Geometry: final body of the model. Coordinates: model frame, mm. A direction names the side the tool comes from. Coordinates: 2 decimals unless noted, no trailing zeros. Write each loop counter-clockwise with the first axis right and the second up, starting at its lowest first coordinate (ties: lowest second). Pieces come first, ordered by that corner, then holes. Notation, with made-up numbers: (20, 2.25) -> (51, 2.25) arc R19 cw to (51, 12.25) -> close; hole circle Ø4 at (77.5, 82.5). An arc over 180 degrees is marked (long way). Answer as a JSON object with one key per item and string values. Group by question number.
```python
from build123d import *

# Parameters (mm, degrees)
F0_W          = 22
F0_H          = 42
F1_DEPTH      = 3
F2_W          = 3
F2_H          = 30
F2_W_2        = 5
F3_DEPTH      = 22
F4_D          = 4.1
F7_DEPTH      = 5
F8_DEPTH      = 2.97
F9_R          = 4.99999
F11_D         = 4.1
F12_D         = 2.8
F13_W         = 22
F13_H         = 10.5
F14_DEPTH     = 8
F15_T1_DEPTH  = 8
F15_T3_DEPTH  = 18
F15_T5_DEPTH  = 18
F15_T7_DEPTH  = 22.7901994578
F15_T9_DEPTH  = 23
F15_T11_DEPTH = 23
F15_T13_DEPTH = 23
F16_D         = 29
F17_D         = 3.1


# Not quite as in the source:
# - a fillet or chamfer that OpenCascade refuses, or shapes differently, is made with other operations: its cross-section is extruded or revolved along the edge and cut away or added
# - a fillet or chamfer is up to 0.001 mm smaller than in the source, because OpenCascade refuses the exact size


with BuildPart() as f1:
    # F0 (on Front) → F1 (new body)
    with BuildSketch(Plane.XZ):
        with Locations((-28.9233987555, 27.9422005266)):
            Rectangle(F0_W, F0_H)
    extrude(amount=F1_DEPTH)

    # F2 (on face) → F3 (join)
    with BuildSketch(Plane(origin=(-39.9233987555, 0, 0), x_dir=(0, -1, 0), z_dir=(-1, 0, 0))):
        with Locations((1.5, 33.9422005266)):
            Rectangle(F2_W, F2_H)
        with Locations((5.5, 33.9422005266)):
            Rectangle(F2_W_2, F2_H)
    extrude(amount=-F3_DEPTH)

    # F4 (through all)
    with Locations(Plane(origin=(0, 0, 0), x_dir=(1, 0, 0), z_dir=(0, 1, 0))):
        with Locations((-24.9233987555, -12.9422005266), (-32.9233987555, -12.9422005266), (-32.9233987555, -32.9422005266), (-24.9233987555, -32.9422005266)):
            Hole(F4_D / 2)

    # F6 (on line) → F7 (join, symmetric)
    with BuildSketch(Plane.XY.offset(23.9422005266)):
        with BuildLine():
            ThreePointArc((-36.9233987555, -20), (-28.9233987555, -12), (-20.9233987555, -20))
            Line((-20.9233987555, -20), (-20.9233987555, -32))
            Line((-20.9233987555, -32), (-17.9233987555, -32))
            Line((-17.9233987555, -32), (-17.9233987555, 0))
            Line((-17.9233987555, 0), (-39.9233987555, 0))
            Line((-39.9233987555, 0), (-39.9233987555, -32))
            Line((-39.9233987555, -32), (-36.9233987555, -32))
            Line((-36.9233987555, -32), (-36.9233987555, -20))
        make_face()
    extrude(amount=F7_DEPTH, both=True)

    # F6 (on line) → F8 (join, symmetric)
    with BuildSketch(Plane.XY.offset(23.9422005266)):
        with BuildLine():
            ThreePointArc((-34.9233987555, -20), (-28.9233987555, -14), (-22.9233987555, -20))
            Line((-22.9233987555, -20), (-22.9233987555, -25.2915026221))
            ThreePointArc((-22.9233987555, -25.2915026221), (-21.4400839819, -22.8284271247), (-20.9233987555, -20))
            ThreePointArc((-20.9233987555, -20), (-28.9233987555, -12), (-36.9233987555, -20))
            ThreePointArc((-36.9233987555, -20), (-36.406713529, -22.8284271247), (-34.9233987555, -25.2915026221))
            Line((-34.9233987555, -25.2915026221), (-34.9233987555, -20))
        make_face()
        with BuildLine():
            Line((-34.9233987555, -32), (-34.9233987555, -25.2915026221))
            ThreePointArc((-34.9233987555, -25.2915026221), (-36.406713529, -22.8284271247), (-36.9233987555, -20))
            Line((-36.9233987555, -20), (-36.9233987555, -32))
            Line((-36.9233987555, -32), (-34.9233987555, -32))
        make_face()
        with BuildLine():
            ThreePointArc((-20.9233987555, -20), (-21.4400839819, -22.8284271247), (-22.9233987555, -25.2915026221))
            Line((-22.9233987555, -25.2915026221), (-22.9233987555, -32))
            Line((-22.9233987555, -32), (-20.9233987555, -32))
            Line((-20.9233987555, -32), (-20.9233987555, -20))
        make_face()
    extrude(amount=F8_DEPTH, both=True)

    # F9 (radius 5 in the source; OpenCascade refuses exactly that, so slightly less here)
    f9_edges = [f1.edges().sort_by_distance(p)[0] for p in [
        (-38.423399, -32, 28.942201),
        (-38.423399, -32, 18.942201),
        (-19.423399, -32, 18.942201),
        (-19.423399, -32, 28.942201),
    ]]
    fillet(f9_edges, radius=F9_R)

    # F11 (through all)
    with Locations(Plane(origin=(-39.9233987555, 0, 0), x_dir=(0, -1, 0), z_dir=(-1, 0, 0))):
        with Locations((4, 44.9422005266), (4, 24.9422005266)):
            Hole(F11_D / 2)

    # F12 (through all)
    with Locations(Plane(origin=(-39.9233987555, 0, 0), x_dir=(0, -1, 0), z_dir=(-1, 0, 0))):
        with Locations((27.5, 23.9422005266)):
            Hole(F12_D / 2)

    # F13 (on Front) → F14 (join)
    with BuildSketch(Plane.XZ):
        Polygon((-57.4233987555, 59.4422005266), (-39.9233987555, 59.4422005266), (-17.9233987555, 59.4422005266), (-15.4233987555, 59.4422005266), (-15.4233987555, 101.4422005266), (-57.4233987555, 101.4422005266), align=None)
        with Locations((-28.9233987555, 54.1922005266)):
            Rectangle(F13_W, F13_H)
    extrude(amount=F14_DEPTH)

    # F15: fillet of radius 3 on 7 edges, made by hand

    # F15_s2 → F15_t1 (join)
    with BuildSketch(Plane.XZ):
        with BuildLine():
            ThreePointArc((-39.9233987555, 56.4422005266), (-40.8020784119, 58.5635208702), (-42.9233987555, 59.4422005266))
            Line((-42.9233987555, 59.4422005266), (-39.9233987555, 59.4422005266))
            Line((-39.9233987555, 59.4422005266), (-39.9233987555, 56.4422005266))
        make_face()
    extrude(amount=F15_T1_DEPTH)

    # F15_s4 → F15_t3 (cut)
    with BuildSketch(Plane.XZ.offset(-7.5)):
        with BuildLine():
            ThreePointArc((-39.9233987555, 9.9422005266), (-39.0447190991, 7.820880183), (-36.9233987555, 6.9422005266))
            Line((-36.9233987555, 6.9422005266), (-39.9233987555, 6.9422005266))
            Line((-39.9233987555, 6.9422005266), (-39.9233987555, 9.9422005266))
        make_face()
    extrude(amount=F15_T3_DEPTH, mode=Mode.SUBTRACT)

    # F15_s6 → F15_t5 (cut)
    with BuildSketch(Plane.XZ.offset(-7.5)):
        with BuildLine():
            ThreePointArc((-17.9233987555, 9.9422005266), (-18.8020784119, 7.820880183), (-20.9233987555, 6.9422005266))
            Line((-20.9233987555, 6.9422005266), (-17.9233987555, 6.9422005266))
            Line((-17.9233987555, 6.9422005266), (-17.9233987555, 9.9422005266))
        make_face()
    extrude(amount=F15_T5_DEPTH, mode=Mode.SUBTRACT)

    # F15_s8 → F15_t7 (cut)
    with BuildSketch(Plane.XZ.offset(-7.3950997289)):
        with BuildLine():
            ThreePointArc((-17.9233987555, 59.4422005266), (-16.132110908, 60.463748745), (-15.4233987555, 62.4002404181))
            Line((-15.4233987555, 62.4002404181), (-15.4233987555, 59.4422005266))
            Line((-15.4233987555, 59.4422005266), (-17.9233987555, 59.4422005266))
        make_face()
    extrude(amount=F15_T7_DEPTH, mode=Mode.SUBTRACT)

    # F15_s10 → F15_t9 (cut)
    with BuildSketch(Plane.XZ.offset(-7.5)):
        with BuildLine():
            ThreePointArc((-18.4233987555, 101.4422005266), (-16.3020784119, 100.5635208702), (-15.4233987555, 98.4422005266))
            Line((-15.4233987555, 98.4422005266), (-15.4233987555, 101.4422005266))
            Line((-15.4233987555, 101.4422005266), (-18.4233987555, 101.4422005266))
        make_face()
    extrude(amount=F15_T9_DEPTH, mode=Mode.SUBTRACT)

    # F15_s12 → F15_t11 (cut)
    with BuildSketch(Plane.XZ.offset(-7.5)):
        with BuildLine():
            ThreePointArc((-57.4233987555, 98.4422005266), (-56.5447190991, 100.5635208702), (-54.4233987555, 101.4422005266))
            Line((-54.4233987555, 101.4422005266), (-57.4233987555, 101.4422005266))
            Line((-57.4233987555, 101.4422005266), (-57.4233987555, 98.4422005266))
        make_face()
    extrude(amount=F15_T11_DEPTH, mode=Mode.SUBTRACT)

    # F15_s14 → F15_t13 (cut)
    with BuildSketch(Plane.XZ.offset(-7.5)):
        with BuildLine():
            ThreePointArc((-54.4233987555, 59.4422005266), (-56.5447190991, 60.320880183), (-57.4233987555, 62.4422005266))
            Line((-57.4233987555, 62.4422005266), (-57.4233987555, 59.4422005266))
            Line((-57.4233987555, 59.4422005266), (-54.4233987555, 59.4422005266))
        make_face()
    extrude(amount=F15_T13_DEPTH, mode=Mode.SUBTRACT)

    # F16 (through all)
    with Locations(Plane(origin=(0, 0, 0), x_dir=(1, 0, 0), z_dir=(0, 1, 0))):
        with Locations((-36.4233987555, -80.4422005266)):
            Hole(F16_D / 2)

    # F17 (through all)
    with Locations(Plane(origin=(0, 0, 0), x_dir=(1, 0, 0), z_dir=(0, 1, 0))):
        with Locations((-51.9233987555, -95.9422005266), (-20.9233987555, -95.9422005266), (-20.9233987555, -64.9422005266), (-51.9233987555, -64.9422005266)):
            Hole(F17_D / 2)


solid = f1.part
```
Item 1: Section A-A on y = -23. Output: boundary loops of the cut face in (x, z).
Item 2: Set-up query: faces 5 (the flat face through (-36.1, -8, 65.7)), 6 (the flat face through (-17.923, -7.6, 30.9)), 7 (the flat face through (-34.923, -26, 25)), 8 (the flat face through (-36, -4, 101.442)), 9 (the flat face through (-29, -3, 13)). Return all of +Z, -Z, +X, -X, +Y, -Y with unobstructed straight access to the full face (end or side cutting, diameter ignored); none if empty.
Item 3: Section D-D on y = -4. Give the number of separate pieces and of enclosed holes in the cut face, then the cut area to 3 significant figures.
Item 4: Ray query, L1, parallel to X at y = -21, z = 27.5; L2, parallel to X at y = -7, z = 80; L3, parallel to Z at x = -36.5, y = -21. Return the intervals inside material, ascending. Write a range as [from, to].
Item 5: Section B-B on x = -24.5. Output: boundary loops of the cut face in (y, z).
Item 6: Mould query, pull axis X, two halves, no side actions, for faces 1 (the flat face through (-29, -11, 28.942)), 2 (the flat face through (-31, -14, 26.912)), 3 (the cylindrical face through (-30.875, -1.521, 12.852)), 4 (the cylindrical face through (-16.33, -3.94, 100.59)). Classes: +X half, -X half, draft (parallel to the pull), parting line (faces both ways), or undercut.
Item 7: Section C-C on z = 92.5. Output: boundary loops of the cut face in (x, y).
Item 8: Contact query for flat-ended pins moving along their axis: pin 1 (8 mm diameter, centred on y = -26, z = 30, fed in from +X); pin 2 (1 mm diameter, centred on y = -10, z = 27.5, fed in from -X); pin 3 (3.5 mm diameter, centred on x = -20.92, z = 95.94, fed in from -Y); pin 4 (3.5 mm diameter, centred on x = -24.92, z = 12.94, fed in from -Y). Output: stop coordinate, or through.
Answer sheet:
{
 "1": {"outline": "(-39.92, 18.94) -> (-36.92, 18.94) -> (-36.92, 20.97) -> (-34.92, 20.97) -> (-34.92, 26.91) -> (-36.92, 26.91) -> (-36.92, 28.94) -> (-39.92, 28.94) -> close; (-22.92, 20.97) -> (-20.92, 20.97) -> (-20.92, 18.94) -> (-17.92, 18.94) -> (-17.92, 28.94) -> (-20.92, 28.94) -> (-20.92, 26.91) -> (-22.92, 26.91) -> close"},
 "2": {"face 5": "+Z, +X, -X, -Y", "face 6": "-Z, +X, +Y, -Y", "face 7": "+Z, -Z, -Y", "face 8": "+Z, +X, -X, +Y, -Y", "face 9": "-Z, +X, -X, -Y"},
 "3": {"separate pieces": "3", "enclosed holes": "7", "area": "1,750 mm^2"},
 "4": {"L1": "x = [-39.92, -36.92], [-20.92, -17.92]", "L2": "x = [-57.42, -50.92], [-21.93, -15.42]", "L3": "z = [20.97, 26.91]"},
 "5": {"outline": "(-15.95, 20.97) -> (-13.33, 20.97) -> (-13.33, 18.94) -> (-3, 18.94) -> (-3, 14.95) -> (0, 14.95) -> (0, 30.94) -> (-8, 30.94) -> (-8, 28.94) -> (-13.33, 28.94) -> (-13.33, 26.91) -> (-15.95, 26.91) -> close; (-8, 34.95) -> (0, 34.95) -> (0, 72.19) -> (-8, 72.19) -> close; (-8, 88.69) -> (0, 88.69) -> (0, 101.44) -> (-8, 101.44) -> close; (-3, 6.94) -> (0, 6.94) -> (0, 10.94) -> (-3, 10.94) -> close; hole circle Ø4.1 at (-4, 24.94); hole circle Ø4.1 at (-4, 44.94)"},
 "6": {"face 1": "draft", "face 2": "undercut", "face 3": "undercut", "face 4": "+X half"},
 "7": {"outline": "(-57.42, -8) -> (-44.48, -8) -> (-44.48, 0) -> (-57.42, 0) -> close; (-28.37, -8) -> (-15.42, -8) -> (-15.42, 0) -> (-28.37, 0) -> close"},
 "8": {"pin 1": "stops at x = -17.92", "pin 2": "stops at x = -39.92", "pin 3": "stops at y = -8", "pin 4": "passes through"}
}
